from build123d import *

# Parameters (mm, degrees)
BOSS_EXTRUDE1_DEPTH = 30


with BuildPart() as part:
    # Sketch1 → Boss-Extrude1 (new body)
    with BuildSketch(Plane.XY):
        with BuildLine():
            Line((-175, -125), (-225, -125))
            ThreePointArc((-225, -125), (-242.67766953, -132.32233047), (-250, -150))
            Line((-250, -150), (-250, -250))
            ThreePointArc((-250, -250), (-242.67766953, -267.67766953), (-225, -275))
            Line((-225, -275), (225, -275))
            ThreePointArc((225, -275), (242.67766953, -267.67766953), (250, -250))
            Line((250, -250), (250, -150))
            ThreePointArc((250, -150), (242.67766953, -132.32233047), (225, -125))
            Line((225, -125), (175, -125))
            ThreePointArc((175, -125), (157.32233047, -117.67766953), (150, -100))
            Line((150, -100), (150, 100))
            ThreePointArc((150, 100), (142.67766953, 117.67766953), (125, 125))
            Line((125, 125), (-125, 125))
            ThreePointArc((-125, 125), (-142.67766953, 117.67766953), (-150, 100))
            Line((-150, 100), (-150, -100))
            ThreePointArc((-150, -100), (-157.32233047, -117.67766953), (-175, -125))
        make_face()
        with BuildLine():
            Line((-20.785894669, 75), (14.336083622, 75))
            ThreePointArc((14.336083622, 75), (34.268791925, 66.743601886), (42.525190039, 46.810893583))
            Line((42.525190039, 46.810893583), (42.525190039, -46.810893583))
            ThreePointArc((42.525190039, -46.810893583), (34.268791925, -66.743601886), (14.336083622, -75))
            Line((14.336083622, -75), (-20.785894669, -75))
            ThreePointArc((-20.785894669, -75), (-40.718602973, -66.743601886), (-48.975001087, -46.810893583))
            Line((-48.975001087, -46.810893583), (-48.975001087, 46.810893583))
            ThreePointArc((-48.975001087, 46.810893583), (-40.718602973, 66.743601886), (-20.785894669, 75))
        make_face(mode=Mode.SUBTRACT)
        with BuildLine():
            Line((-100.16408543, -174.707408676), (99.83591457, -174.707408676))
            ThreePointArc((99.83591457, -174.707408676), (124.917346487, -199.625710645), (99.999044519, -224.707142562))
            Line((99.999044519, -224.707142562), (-105.412874128, -224.707142562))
            ThreePointArc((-105.412874128, -224.707142562), (-125.154899456, -197.359330907), (-100.16408543, -174.707408676))
        make_face(mode=Mode.SUBTRACT)
    extrude(amount=BOSS_EXTRUDE1_DEPTH)


solid = part.part
Can you work these out from the model? Positions are in its coordinate system, mm. A direction names the side the tool comes from. Round coordinates to 2 decimals unless told otherwise and drop trailing zeros. Write each loop counter-clockwise with the first axis right and the second up, starting at its lowest first coordinate (ties: lowest second). Pieces come first, ordered by that corner, then holes. Notation, with made-up numbers: (59, -21) -> (70, -21) arc R26 ccw to (70, 17) -> close; hole circle Ø5 at (28, 76.5). An arc over 180 degrees is marked (long way). One line per question, with ' | ' between items. Start each with the question number.
1) I need wall thicknesses on line 1 (Y direction, x = -14, z = 7.25); line 2 (Y direction, x = -77, z = 18); line 3 (X direction, y = 21.5, z = 27.5) (3 decimals). Which ranges of each line are inside material? Lowest first, please. Write a range as [from, to].
2) Suppose I cut it at D-D on y = -52. Write out the boundary of the cut face in (x, z).
3) I'm going to push flat-ended pins straight in: P1, Ø9, axis at x = -192.5, z = 7.5, coming from the +Y side; P2, Ø15, axis at y = 8, z = 15, coming from the -X side; P3, Ø6, axis at x = 144, z = 18, coming from the +Y side. Where does each tip first touch, or does it pass through?
4) Suppose I cut it at C-C on z = 5.5. Write out the boundary of the cut face in (x, y) (3 decimals).
5) If we mould it in two halves opening along X, with no side actions, what happens to faces 4 (the cylindrical face through (-242.871, -267.482, 14.79)), 5 (the flat face through (-2, -174.707, 15)), 6 (the flat face through (2, 125, 15))? For each: released by +X, released by -X, zero draft, split by the parting line, or undercut.
6) Suppose I cut it at A-A on y = 12.5. Write out the boundary of the cut face in (x, z) (3 decimals).
7) Suppose I cut it at B-B on x = -1. Write out the boundary of the cut face in (y, z).
8) On a 3-axis mill with a long thin cutter (end or side, diameter ignored), from which of +Z, -Z, +X, -X, +Y, -Y can I reach the whole of each face in a straight line? I mean faces 1 (the flat face through (-3, -275, 15)), 2 (the flat face through (-3, -75, 15)), 3 (the flat face through (-200, -125, 15)). Say none if no direction works.
Return value:
1) line 1: y = [-275, -224.71], [-174.71, -75], [75, 125] | line 2: y = [-275, -224.71], [-174.71, 125] | line 3: x = [-150, -48.975], [42.525, 150]
2) outline: (-150, 0) -> (-48.49, 0) -> (-48.49, 30) -> (-150, 30) -> close; (42.04, 0) -> (150, 0) -> (150, 30) -> (42.04, 30) -> close
3) P1: stops at y = -125 | P2: stops at x = -150 | P3: stops at y = 119.21
4) outline: (-250, -250) arc R25 ccw to (-225, -275) -> (225, -275) arc R25 ccw to (250, -250) -> (250, -150) arc R25 ccw to (225, -125) -> (175, -125) arc R25 cw to (150, -100) -> (150, 100) arc R25 ccw to (125, 125) -> (-125, 125) arc R25 ccw to (-150, 100) -> (-150, -100) arc R25 cw to (-175, -125) -> (-225, -125) arc R25 ccw to (-250, -150) -> close; hole (-105.413, -224.707) -> (99.999, -224.707) arc R25 ccw to (99.836, -174.707) -> (-100.164, -174.707) arc R25.293 ccw to start; hole (-48.975, -46.811) arc R28.189 ccw to (-20.786, -75) -> (14.336, -75) arc R28.189 ccw to (42.525, -46.811) -> (42.525, 46.811) arc R28.189 ccw to (14.336, 75) -> (-20.786, 75) arc R28.189 ccw to (-48.975, 46.811) -> close
5) face 4: released by -X | face 5: undercut | face 6: zero draft
6) outline: (-150, 0) -> (-48.975, 0) -> (-48.975, 30) -> (-150, 30) -> close; (42.525, 0) -> (150, 0) -> (150, 30) -> (42.525, 30) -> close
7) outline: (-275, 0) -> (-224.71, 0) -> (-224.71, 30) -> (-275, 30) -> close; (-174.71, 0) -> (-75, 0) -> (-75, 30) -> (-174.71, 30) -> close; (75, 0) -> (125, 0) -> (125, 30) -> (75, 30) -> close
8) face 1: +Z, -Z, +X, -X, -Y | face 2: +Z, -Z | face 3: +Z, -Z, -X, +Y
